Build history of the part. All positions in model axes, mm. Round coordinates to 2 decimals unless told otherwise and drop trailing zeros. Loops run counter-clockwise (first coordinate to the right, second up) from the corner with the lowest first, then second, coordinate; pieces in that order, holes last. Notation, with made-up numbers: (27.5, 5.5) - (81.5, 5.5) arc R22 cw to (81.5, 40.5) - close; hole circle Ø10 at (72, 31.25). An arc over 180 degrees is marked (long way). Use a Markdown table: item, result.
from build123d import *

# Parameters (mm, degrees)
F0_W          = 375.5
F0_H          = 10
F1_DEPTH      = 1825.5
F2_T          = -2.5
F3_R          = 2
F4_DEPTH      = 20
F4_DEPTH_BACK = 1835
F5_R          = 12.88095
F6_DEPTH      = 5
F7_R          = 26.336988
F8_DEPTH      = 25
F9_R          = 5
F10_W         = 17.191563
F10_H         = 6.224573
F11_DEPTH     = 5


with BuildPart() as f1:
    # F0 (on Top) → F1 (new body)
    with BuildSketch(Plane.XY):
        with Locations((187.75, 5)):
            Rectangle(F0_W, F0_H)
    extrude(amount=F1_DEPTH)

    # F2
    f2_openings = [f1.faces().sort_by_distance(p)[0] for p in [
        (187.75, 10, 912.75),
    ]]
    offset(amount=F2_T, openings=f2_openings)

    # F3 (on face) → F4 (join, two sides)
    with BuildSketch(Plane(origin=(0, 0, 0), x_dir=(1, 0, 0), z_dir=(0, 0, -1))) as f4_sk:
        with Locations((366.5, -5)):
            Circle(F3_R)
    extrude(amount=F4_DEPTH)
    extrude(f4_sk.sketch, amount=-F4_DEPTH_BACK)

    # F5 (on face) → F6 (join)
    with BuildSketch(Plane.XZ):
        with Locations((36.467917, 900.125802)):
            Circle(F5_R)
    extrude(amount=F6_DEPTH)

    # F7 (on face) → F8 (join)
    with BuildSketch(Plane.XZ.offset(5)):
        with Locations((36.467917, 900.125802)):
            Circle(F7_R)
    extrude(amount=F8_DEPTH)

    # F9
    f9_edges = [f1.edges().sort_by_distance(p)[0] for p in [
        (10.130929, -30, 900.125802),
        (10.130929, -5, 900.125802),
    ]]
    fillet(f9_edges, radius=F9_R)

    # F10 (on face) → F11 (cut)
    with BuildSketch(Plane.XZ.offset(30)):
        with Locations((35.949202, 900.496275)):
            Rectangle(F10_W, F10_H)
    extrude(amount=-F11_DEPTH, mode=Mode.SUBTRACT)


solid = f1.part
Q1. Cut at A-A, the plane z = 965.5. List the corners of the cut face in (x, y).
Results found:
| item | result |
|---|---|
| outline | (0, 0) - (375.5, 0) - (375.5, 10) - (373, 10) - (373, 2.5) - (2.5, 2.5) - (2.5, 10) - (0, 10) - close; circle Ø4 at (366.5, 5) |
Q2. Cut at C-C, the plane y = -19. List the corners of the cut face in (x, z), plus the area to 3 significant figures.
Results found:
| item | result |
|---|---|
| outline | circle Ø52.67 at (36.47, 900.13) |
| area | 2,180 mm2 |
Q3. Pull direction X, two halves, no side cores. Call faces 1 (the face through (185, 2.5, 900)), 2 (the face through (33.04, -17.4, 926.24)), 3 (the face through (46, -5, 891)): pulls with the +X half, pulls with the -X half, needs draft (parallel to the pull), parting line crosses it, or undercut.
Results found:
| item | result |
|---|---|
| face 1 | undercut |
| face 2 | parting line crosses it |
| face 3 | needs draft |
Q4. Probe line 1 (X direction, y = 6, z = 595); line 2 (Z direction, x = 155, y = 3); line 3 (Y direction, x = 347.5, z = 187). List the from-to ranges inside material, lowest first.
Results found:
| item | result |
|---|---|
| line 1 | x = 0 to 2.5, 364.77 to 368.23, 373 to 375.5 |
| line 2 | z = 0 to 2.5, 1823 to 1825.5 |
| line 3 | y = 0 to 2.5 |
Q5. Cut at B-B, the plane x = 321. List the corners of the cut face in (y, z).
Results found:
| item | result |
|---|---|
| outline | (0, 0) - (10, 0) - (10, 2.5) - (2.5, 2.5) - (2.5, 1823) - (10, 1823) - (10, 1825.5) - (0, 1825.5) - close |
Q6. Drop flat-ended pins along their axis: pin 1 (11 mm diameter, centred on x = 260.5, y = 6, fed in from -Z); pin 2 (2.5 mm diameter, centred on x = 34, y = -27, fed in from -Z); pin 3 (1.5 mm diameter, centred on x = 34, y = -28.5, fed in from +Z); pin 4 (6 mm diameter, centred on x = 81, y = -4, fed in from -Z). Give the stop position or say it passes through.
Results found:
| item | result |
|---|---|
| pin 1 | stops at z = 0 |
| pin 2 | stops at z = 873.94 |
| pin 3 | stops at z = 925.52 |
| pin 4 | passes through |
